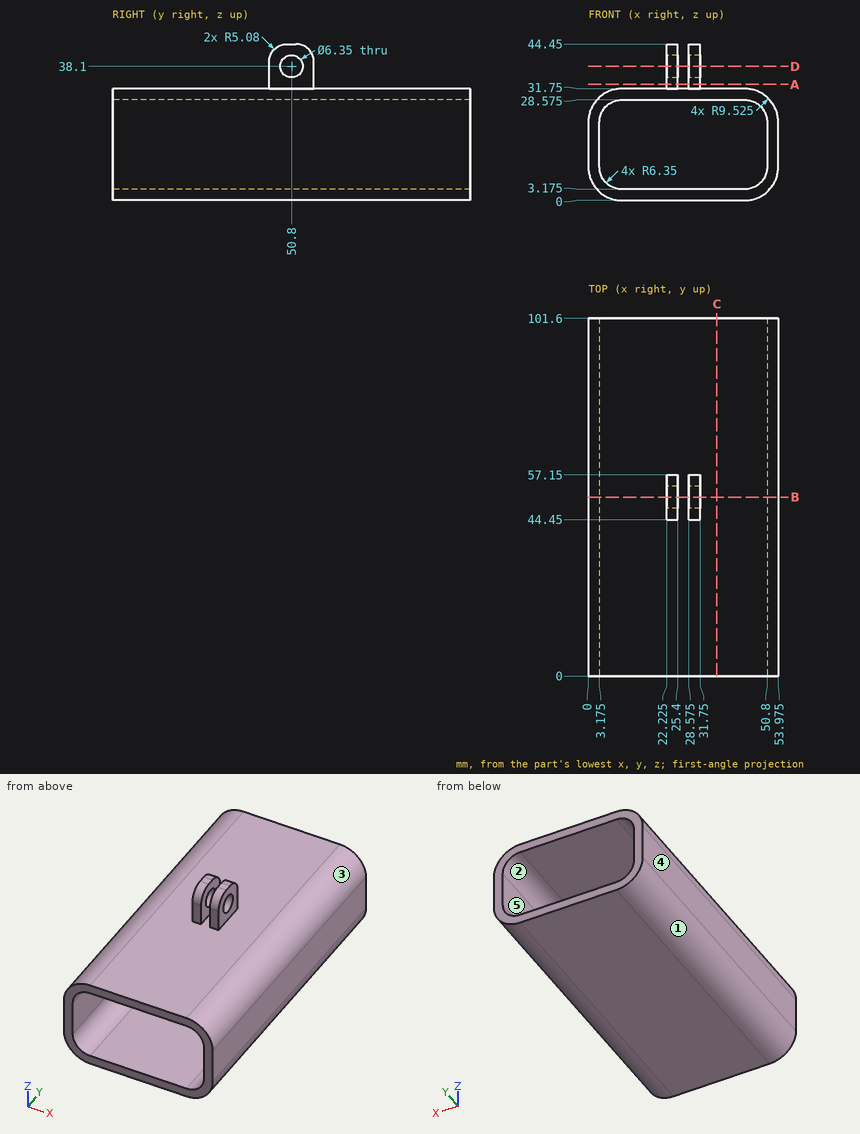
Print and shaded views of the part. All mm, measured from the part's lowest x, y and z. A direction names the side the tool comes from. Round coordinates to 2 decimals unless told otherwise and drop trailing zeros. Write each loop counter-clockwise with the first axis right and the second up, starting at its lowest first coordinate (ties: lowest second). Pieces come first, ordered by that corner, then holes. Notation, with made-up numbers: M 0,40.25 L 53,40.25 A19 ccw 53,56.25 Z; hole C 13.25,75.25 d5. An arc over 180 degrees is marked long. One line per question, with ' | ' between items.
(1) Saw through at B-B on y = 50.8. Count the separate pieces of the cut face and the enclosed holes in it, then the cut area to 3 significant figures.
Answer key:
separate pieces: 3 | enclosed holes: 1 | area: 501 mm^2
(2) Saw through at C-C on x = 36.5. Write the cut outline in (y, z) (3 decimals), then the cut area to 3 significant figures.
Answer key:
outline: M 0,0 L 101.6,0 L 101.6,3.175 L 0,3.175 Z; M 0,28.575 L 101.6,28.575 L 101.6,31.75 L 0,31.75 Z | area: 645 mm^2
(3) Probe line 1 along X through (y, z) = (74, 12.5) (3 decimals); line 2 along Z through (x, y) = (37.5, 80) (3 decimals); line 3 along Z through (x, y) = (31, 50) (3 decimals). List the from-to ranges inside material, lowest first.
Answer key:
line 1: x = 0 to 3.175, 50.8 to 53.975 | line 2: z = 0 to 3.175, 28.575 to 31.75 | line 3: z = 0 to 3.175, 28.575 to 35.027, 41.173 to 44.45
(4) 3-axis set-ups, long thin cutter, end or side, ignore diameter. For the marked faces 4 and 5: which of +Z, -Z, +X, -X, +Y, -Y reach the whole face in a straight line?
Answer key:
face 4: +Z, -Z, -X, +Y, -Y | face 5: +Y, -Y
(5) Two-plate mould, pull along X, no slides. Class the marked faces 1, 2 and 3: released by +X, released by -X, zero draft, split by the parting line, or undercut.
Answer key:
face 1: released by -X | face 2: undercut | face 3: released by +X
(6) Saw through at A-A on z = 33. Write the cut outline in (x, y) (3 decimals).
Answer key:
outline: M 22.225,44.45 L 25.4,44.45 L 25.4,57.15 L 22.225,57.15 Z; M 28.575,44.45 L 31.75,44.45 L 31.75,57.15 L 28.575,57.15 Z
(7) Saw through at D-D on z = 38.1. Write the cut outline in (x, y) (3 decimals).
Answer key:
outline: M 22.225,44.45 L 25.4,44.45 L 25.4,47.625 L 22.225,47.625 Z; M 22.225,53.975 L 25.4,53.975 L 25.4,57.15 L 22.225,57.15 Z; M 28.575,44.45 L 31.75,44.45 L 31.75,47.625 L 28.575,47.625 Z; M 28.575,53.975 L 31.75,53.975 L 31.75,57.15 L 28.575,57.15 Z
(8) Pin check, flat tips, straight feed: pin 1 (4 mm diameter, centred on y = 48.5, z = 38, fed in from -X) (3 decimals); pin 2 (17.5 mm diameter, centred on x = 32.5, y = 26.5, fed in from +Z); pin 3 (2.5 mm diameter, centred on x = 23.5, z = 34.5, fed in from +Y); pin 4 (4 mm diameter, centred on y = 50.8, z = 38.1, fed in from +X). Stop position of each tip, or through.
Answer key:
pin 1: stops at x = 22.225 | pin 2: stops at z = 31.75 | pin 3: stops at y = 57.15 | pin 4: passes through
